Geometry: see drawing. Coordinates: mm, zero at the bounding-box minimum. A direction names the side the tool comes from. Coordinates: 2 decimals unless noted, no trailing zeros. Write each loop counter-clockwise with the first axis right and the second up, starting at its lowest first coordinate (ties: lowest second). Pieces come first, ordered by that corner, then holes. Notation, with made-up numbers: (-4, 15.5) -> (29, 15.5) arc R18 cw to (29, 30.5) -> close; hole circle Ø10 at (81.5, 86). An arc over 180 degrees is marked (long way). Use one line per item in the form item = value. Start each with the question number.
(1) Cut plane D-D on y = 48. Return the cut outline in (x, z).
(2) Pull-direction query (X, two-part tool) for the marked faces 4, 5 and 6; classes: released by +X, released by -X, zero draft, split by the parting line, or undercut.
(3) First-contact query: pin 1 (5 mm diameter, centred on y = 19.5, z = 18, fed in from +X); pin 2 (6 mm diameter, centred on x = 33, z = 21, fed in from -Y). Flat tips, straight axial feed; report the tip coordinate or a pass-through.
(4) Set-up query: the marked faces 1, 2 and 3. Return all of +Z, -Z, +X, -X, +Y, -Y with unobstructed straight access to the full face (end or side cutting, diameter ignored); none if empty.
(5) Cut plane C-C on x = 14. Return the cut outline in (y, z), plus the area to 4 significant figures.
(6) Cut plane A-A on y = 58. Return the cut outline in (x, z), plus the area to 3 significant figures.
(7) Ray query, line 1 along Z through (x, y) = (16, 60.5); line 2 along X through (y, z) = (17.5, 12); line 3 along Y through (x, z) = (78.5, 10.25). Return the intervals inside material, ascending.
(8) Cut plane B-B on z = 5.75. Return the cut outline in (x, y), plus the area to 3 significant figures.
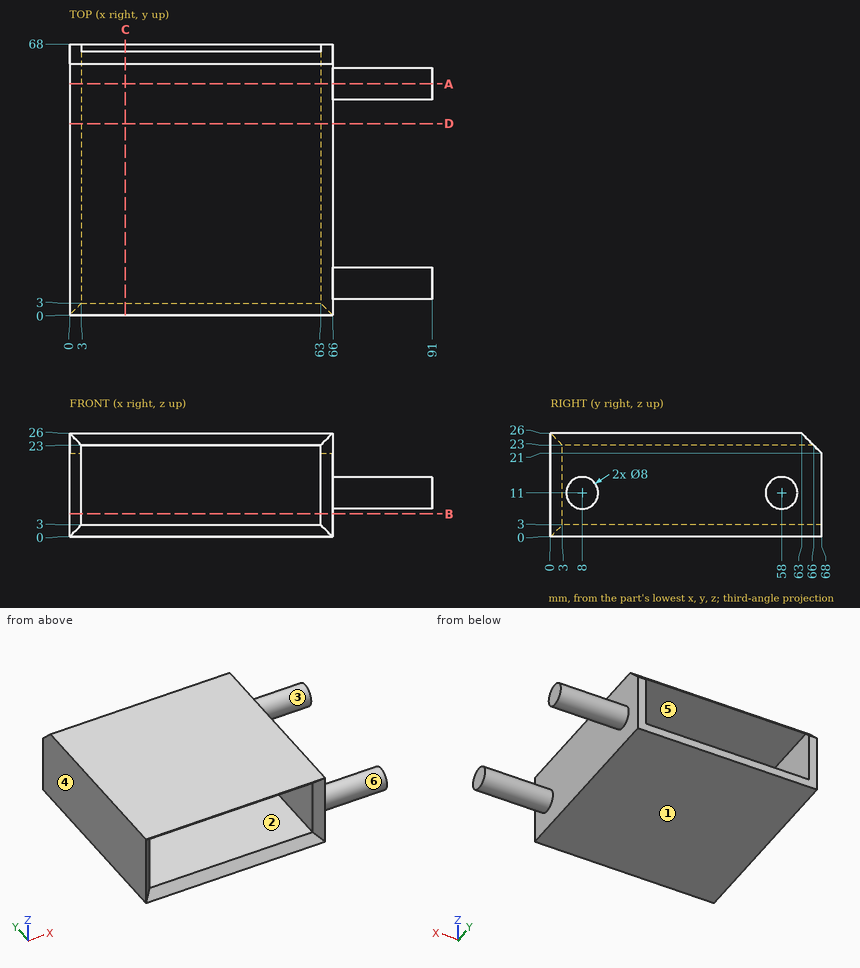
Values:
q1.outline = (0, 0) -> (66, 0) -> (66, 26) -> (0, 26) -> close; hole (3, 3) -> (63, 3) -> (63, 23) -> (3, 23) -> close
q2.face_4 = released by -X
q2.face_5 = undercut
q2.face_6 = zero draft
q3.pin_1 = 66
q3.pin_2 = 2
q4.face_1 = -Z, +X, -X, +Y, -Y
q4.face_2 = +Y, -Y
q4.face_3 = +X
q5.outline = (0, 0) -> (68, 0) -> (68, 3) -> (3, 3) -> close; (0, 26) -> (3, 23) -> (66, 23) -> (63, 26) -> close
q5.area = 388.5 mm2
q6.outline = (0, 0) -> (66, 0) -> (66, 7) -> (91, 7) -> (91, 15) -> (66, 15) -> (66, 26) -> (0, 26) -> close; hole (3, 3) -> (63, 3) -> (63, 23) -> (3, 23) -> close
q6.area = 716 mm2
q7.line_1 = 0 to 3, 23 to 26
q7.line_2 = 0 to 3, 63 to 66
q7.line_3 = 4.07 to 11.93, 54.07 to 61.93
q8.outline = (0, 0) -> (3, 3) -> (3, 68) -> (0, 68) -> close; (63, 3) -> (66, 0) -> (66, 68) -> (63, 68) -> close
q8.area = 399 mm2
